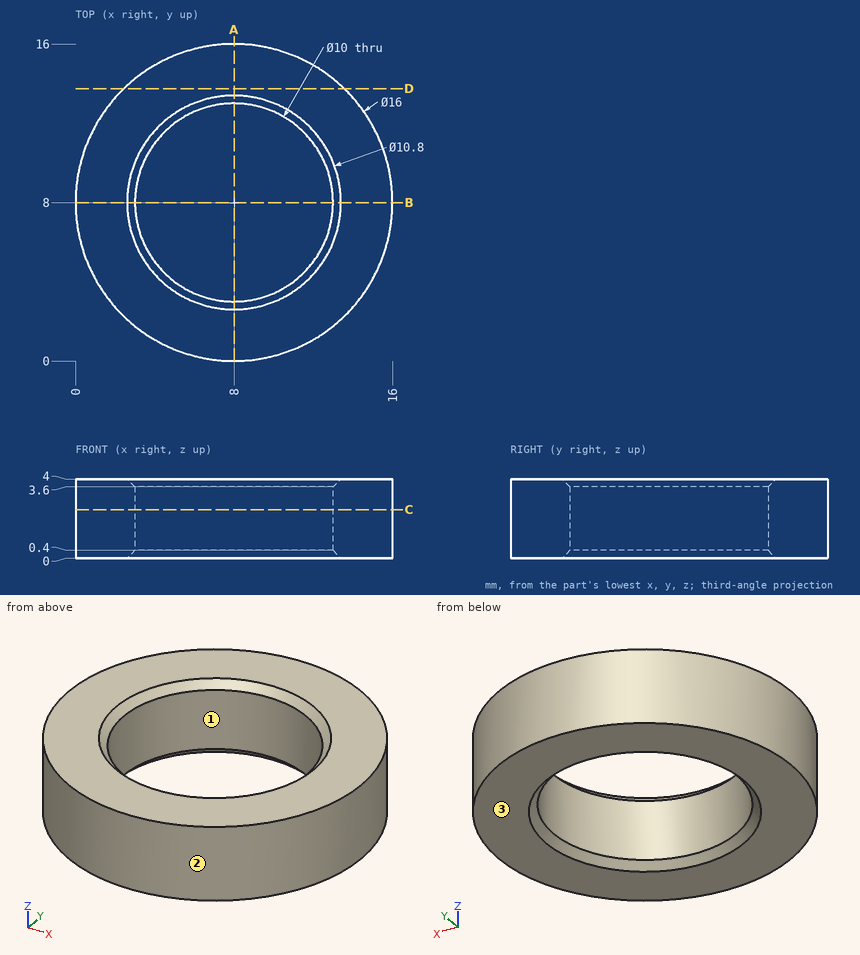
Design review of the part shown in the three views and the two pictorial views. Dimensions are in mm from the part's minimum x, y and z. Round coordinates to 2 decimals unless told otherwise and drop trailing zeros. Loops run counter-clockwise (first coordinate to the right, second up) from the corner with the lowest first, then second, coordinate; pieces in that order, holes last. Notation, with made-up numbers: (-11.75, -39) -> (31.25, -39) arc R33 ccw to (31.25, -6) -> close; hole circle Ø1 at (14, 60). An arc over 180 degrees is marked (long way). Answer as a JSON object with one key per item and string values. Group by question number.
1) For line 1 (Y direction, x = 8, z = 1.5); line 2 (Y direction, x = 4.5, z = 2.45); line 3 (X direction, y = 3.5, z = 0.9), list the stretches that pass through material, from the lowest coordinate up. Write a range as [from, to].
2) We need section C-C on z = 2.45. Write out the cut boundary in (x, y), then the cut area to 3 significant figures.
3) For pin 1 Ø1 at (y, z) = (11, 1) entering from +X; pin 2 Ø8 at (x, y) = (7.5, 7) entering from +Z; pin 3 Ø1.5 at (x, y) = (11, 11.5) entering from +Z, all flat-tipped, find the tip position at first contact; note any pin that passes through.
4) We need section D-D on y = 13.75. Write out the cut boundary in (x, z).
5) Mouldability with a two-part tool opening along X and no side actions: class the marked faces 1, 2 and 3 as released by +X, released by -X, zero draft, split by the parting line, or undercut.
6) We need section A-A on x = 8. Write out the cut boundary in (y, z), then the cut area to 3 significant figures.
Result set:
{
 "1": {"line 1": "[0, 3], [13, 16]", "line 2": "[0.81, 4.43], [11.57, 15.19]", "line 3": "[1.39, 5.82], [10.18, 14.61]"},
 "2": {"outline": "circle Ø16 at (8, 8); hole circle Ø10 at (8, 8)", "area": "123 mm²"},
 "3": {"pin 1": "x = 15.6", "pin 2": "z = 3.72", "pin 3": "z = 3.96"},
 "4": {"outline": "(2.44, 0) -> (13.56, 0) -> (13.56, 4) -> (2.44, 4) -> close"},
 "5": {"face 1": "undercut", "face 2": "split by the parting line", "face 3": "zero draft"},
 "6": {"outline": "(0, 0) -> (2.6, 0) -> (3, 0.4) -> (3, 3.6) -> (2.6, 4) -> (0, 4) -> close; (13, 0.4) -> (13.4, 0) -> (16, 0) -> (16, 4) -> (13.4, 4) -> (13, 3.6) -> close", "area": "23.7 mm²"}
}
